Verification items for the finished model (mm, model axes). A direction names the side the tool comes from. Round coordinates to 2 decimals unless told otherwise and drop trailing zeros. Write each loop counter-clockwise with the first axis right and the second up, starting at its lowest first coordinate (ties: lowest second). Pieces come first, ordered by that corner, then holes.
from build123d import *

# Parameters (mm, degrees)
F0_W     = 210
F0_H     = 125
F1_DEPTH = 6.4
F3_DEPTH = 25
F5_DEPTH = 6.401
F6_SIZE  = 10
F7_W     = 69
F7_H     = 95
F8_DEPTH = 6.401
F9_SIZE  = 10


with BuildPart() as f1:
    # F0 (on Top) → F1 (new body)
    with BuildSketch(Plane.XY):
        Rectangle(F0_W, F0_H)
    extrude(amount=F1_DEPTH)

    # F2 (on face) → F3 (cut)
    with BuildSketch(Plane.XY.offset(6.4)):
        Polygon((105, 10.5), (51, 10.5), (47.755322, 9.986093), (44.828255, 8.494678), (42.505322, 6.171745), (41.013907, 3.244678), (40.5, 0), (41.013907, -3.244678), (42.505322, -6.171745), (44.828255, -8.494678), (47.755322, -9.986093), (51, -10.5), (105, -10.5), align=None)
    extrude(amount=-F3_DEPTH, mode=Mode.SUBTRACT)

    # F4 (on Top) → F5 (cut, through all)
    with BuildSketch(Plane.XY):
        Polygon((89.661921, 53.473939), (90, 53.37467), (90.338079, 53.473939), (90.56882, 53.740228), (90.618965, 54.088994), (90.472593, 54.409504), (90.176176, 54.6), (89.823824, 54.6), (89.527407, 54.409504), (89.381035, 54.088994), (89.43118, 53.740228), align=None)
        Polygon((90.472593, -54.409504), (90.618965, -54.088994), (90.56882, -53.740228), (90.338079, -53.473939), (90, -53.37467), (89.661921, -53.473939), (89.43118, -53.740228), (89.381035, -54.088994), (89.527407, -54.409504), (89.823824, -54.6), (90.176176, -54.6), align=None)
        Polygon((-0.62918, 53.48961), (-0.4, 53.805048), (-0.4, 54.194952), (-0.62918, 54.51039), (-1, 54.630877), (-1.37082, 54.51039), (-1.6, 54.194952), (-1.6, 53.805048), (-1.37082, 53.48961), (-1, 53.369123), align=None)
        Polygon((-1.37082, -53.48961), (-1.6, -53.805048), (-1.6, -54.194952), (-1.37082, -54.51039), (-1, -54.630877), (-0.62918, -54.51039), (-0.4, -54.194952), (-0.4, -53.805048), (-0.62918, -53.48961), (-1, -53.369123), align=None)
    extrude(amount=F5_DEPTH, mode=Mode.SUBTRACT)

    # F6
    f6_edges = [f1.edges().sort_by_distance(p)[0] for p in [
        (-105, 62.5, 3.2),
        (105, 62.5, 3.2),
        (105, -62.5, 3.2),
        (-105, -62.5, 3.2),
    ]]
    chamfer(f6_edges, length=F6_SIZE)

    # F7 (on face) → F8 (cut, through all)
    with BuildSketch(Plane(origin=(0, 0, 0), x_dir=(1, 0, 0), z_dir=(0, 0, -1))):
        with Locations((-50.5, 0)):
            Rectangle(F7_W, F7_H)
    extrude(amount=-F8_DEPTH, mode=Mode.SUBTRACT)

    # F9
    f9_edges = [f1.edges().sort_by_distance(p)[0] for p in [
        (-85, 47.5, 3.2),
        (-16, 47.5, 3.2),
        (-16, -47.5, 3.2),
        (-85, -47.5, 3.2),
    ]]
    chamfer(f9_edges, length=F9_SIZE)


solid = f1.part
Q1. Material ranges on line 1 along X through (y, z) = (14, 4.25); line 2 along Y through (x, z) = (-34.5, 2); line 3 along Y through (x, z) = (48, 1.25), recorded low to high.
Recorded:
line 1: x = -105 to -85, -16 to 105
line 2: y = -62.5 to -47.5, 47.5 to 62.5
line 3: y = -62.5 to -10.02, 10.02 to 62.5
Q2. Tool access check on faces 1 (the flat face through (-16, 1, 3)), 2 (the flat face through (78, -10.5, 3)), 3 (the flat face through (22, 1, 6.4)). Record the directions out of +Z, -Z, +X, -X, +Y, -Y that give a thin tool (end or side, any length) a straight path to the whole face; none if there is none.
Recorded:
face 1: +Z, -Z
face 2: +Z, -Z, +X
face 3: +Z, +X, -X, +Y, -Y
Q3. Depth check by flat-ended pin: P1, Ø3, axis at x = -10, y = -16.5, coming from the -Z side. Enter the tip coordinate at first touch or a pass-through.
Recorded:
P1: stops at z = 0
Q4. Release check for a two-part mould opening along Y. For faces 4 (the flat face through (-1, 62.5, 3)), 5 (the flat face through (105, -32, 3)), 6 (the flat face through (-21.1, 42.6, 3.2)) record: released by +Y, released by -Y, zero draft, split by the parting line, or undercut.
Recorded:
face 4: released by +Y
face 5: zero draft
face 6: undercut
Q5. Sectioned sample at B-B (y = -20.5). Enter the section's corners in (x, z).
Recorded:
outline: (-105, 0) - (-85, 0) - (-85, 6.4) - (-105, 6.4) - close; (-16, 0) - (105, 0) - (105, 6.4) - (-16, 6.4) - close
Q6. Sectioned sample at C-C (z = 4.5). Give the number of separate pieces and of enclosed holes in the cut face, plus the area to 3 significant figures.
Recorded:
separate pieces: 1
enclosed holes: 5
area: 18,400 mm2
Q7. Sectioned sample at A-A (x = 55). Enter the section's corners in (y, z), plus the area to 3 significant figures.
Recorded:
outline: (-62.5, 0) - (-10.5, 0) - (-10.5, 6.4) - (-62.5, 6.4) - close; (10.5, 0) - (62.5, 0) - (62.5, 6.4) - (10.5, 6.4) - close
area: 666 mm2
